Can you work these out from the drawing? Everything is in mm from the part's minimum corner. Give positions to 0.01 mm unless a question says otherwise; leave off trailing zeros. Order: outer loops, then holes, each group sorted by start corner. A loop starts at its lowest first (then second) coordinate and runs counter-clockwise, first axis right, second up. Notation, with made-up numbers: (-4, 71.25) - (42, 71.25) arc R22 ccw to (42, 101.25) - close; hole circle Ø5 at (44.5, 12). An arc over 180 degrees is marked (long way). Answer as a JSON object with one key per item and string values.
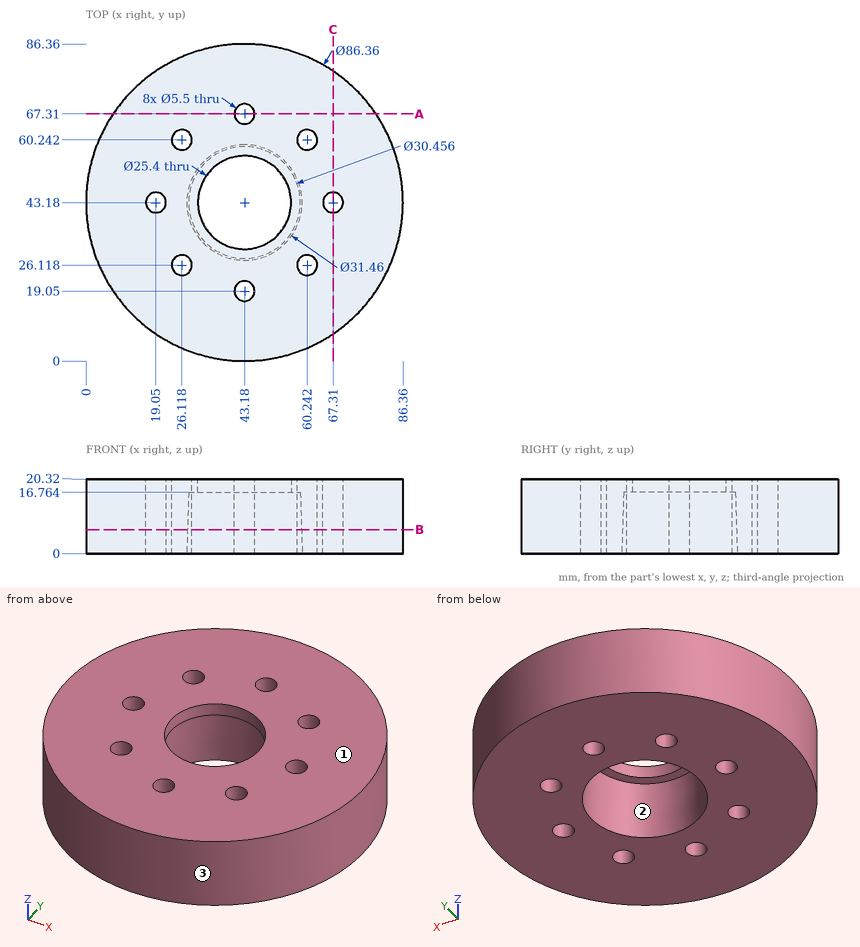
Q1. If we section it at A-A, the plane y = 67.31: Please give me the cut outline in (x, z), then the cut area to 3 significant figures.
Recorded:
{"outline": "(7.37, 0) - (40.43, 0) - (40.43, 20.32) - (7.37, 20.32) - close; (45.93, 0) - (78.99, 0) - (78.99, 20.32) - (45.93, 20.32) - close", "area": "1,340 mm^2"}
Q2. I'm going to push flat-ended pins straight in: pin 1 Ø4.5 at (x, y) = (67.31, 43.18) entering from -Z; pin 2 Ø6 at (x, z) = (37, 12.5) entering from +Y; pin 3 Ø8 at (x, z) = (47.5, 17.5) entering from -Y; pin 4 Ø10 at (x, z) = (63.5, 4) entering from -Y. Where does each tip first touch, or does it pass through?
Recorded:
{"pin 1": "passes through", "pin 2": "stops at y = 86.24", "pin 3": "stops at y = 0", "pin 4": "stops at y = 2.81"}
Q3. If we section it at B-B, the plane z = 6.5: Count the separate pieces of the cut face and the enclosed holes in it, then the cut area to 3 significant figures.
Recorded:
{"separate pieces": "1", "enclosed holes": "9", "area": "4,910 mm^2"}
Q4. I need wall thicknesses on L1, parallel to Y at x = 43.18, z = 5.5 (1 decimal); L2, parallel to X at y = 62, z = 16.5 (1 decimal); L3, parallel to Y at x = 43.18, z = 4. Which ranges of each line are inside material? Lowest first, please.
Recorded:
{"L1": "y = 0 to 16.3, 21.8 to 27.6, 58.7 to 64.6, 70.1 to 86.4", "L2": "x = 4.3 to 24, 28.2 to 58.1, 62.4 to 82", "L3": "y = 0 to 16.3, 21.8 to 27.57, 58.79 to 64.56, 70.06 to 86.36"}
Q5. We'd pull the mould along X, two halves only. Please class the marked faces 1, 2 and 3: released by +X, released by -X, zero draft, split by the parting line, or undercut.
Recorded:
{"face 1": "zero draft", "face 2": "undercut", "face 3": "split by the parting line"}
